Design review of the part built by this model. Coordinates are the model's own, in mm. A direction names the side the tool comes from. Round coordinates to 2 decimals unless told otherwise and drop trailing zeros. Loops run counter-clockwise (first coordinate to the right, second up) from the corner with the lowest first, then second, coordinate; pieces in that order, holes last. Notation, with made-up numbers: (69.25, 55.25) - (128.25, 55.25) arc R13 cw to (128.25, 69.25) - close; hole circle Ø5 at (45, 45). An arc over 180 degrees is marked (long way). Return JSON: item names as keys, results as strings. Group by question number.
(1) Wall thickness on L1, parallel to Y at x = 2, z = 2.1; L2, parallel to Y at x = 0.25, z = 3.8; L3, parallel to X at y = 2, z = 3.6 (3 decimals): over which ranges is each line inside the solid? List them lowest first. Write a range as [from, to].
(2) We need section D-D, the plane x = 10. Write out the cut boundary in (y, z), and give its area (3 significant figures).
(3) For faces 5 (the flat face through (4, 0, 4)), 6 (the flat face through (2.5, 0, 2)), list the 3-axis set-ups (+Z, -Z, +X, -X, +Y, -Y) from which the entire face can be reached by the end or side of a thin tool; tool diameter is ignored.
(4) We need section A-A, the plane x = 6.75. Write out the cut boundary in (y, z), and give its area (3 significant figures).
(5) The part is to be moulded in two halves that separate along X. For faces 1 (the flat face through (8, -2.5, 2)), 2 (the cylindrical face through (-3.75, -0.08, 1.97)), 3 (the flat face through (4, -3.75, 2)), 4 (the flat face through (6, -1, 2)), say which applies: pulls with the +X half, pulls with the -X half, needs draft (parallel to the pull), parting line crosses it, or undercut.
(6) We need section C-C, the plane z = 0.3. Write out the cut boundary in (x, y) (3 decimals), and give its area (3 significant figures).
(7) We need section B-B, the plane y = 0. Write out the cut boundary in (x, z) (3 decimals).
(8) Clearance check with flat-ended pins moving along their axes: pin 1 (1 mm diameter, centred on x = 9, z = 0.5, fed in from -Y); pin 2 (1.2 mm diameter, centred on y = -2, z = 1.5, fed in from +X); pin 3 (1.2 mm diameter, centred on y = 1.5, z = 1, fed in from +X). State where each tip first meets the part, or that it passes through.
from build123d import *

# Parameters (mm, degrees)
BOSS_EXTRUDE1_DEPTH = 4


with BuildPart() as part:
    # Sketch1 → Boss-Extrude1 (new body)
    with BuildSketch(Plane.XY):
        with BuildLine():
            Line((0, 3.75), (8.125, 3.75))
            ThreePointArc((8.125, 3.75), (11.875, 0), (8.125, -3.75))
            Line((8.125, -3.75), (0, -3.75))
            ThreePointArc((0, -3.75), (-3.75, 0), (0, 3.75))
        make_face()
        Polygon((8.125, 2.5), (9.125, 2.5), (9.125, 1), (10.625, 1), (10.625, -1), (9.125, -1), (9.125, -2.5), (7.125, -2.5), (7.125, -1), (5.625, -1), (5.625, 1), (7.125, 1), (7.125, 2.5), align=None, mode=Mode.SUBTRACT)
        Polygon((1, 1), (1, 2.5), (0, 2.5), (-1, 2.5), (-1, 1), (-2.5, 1), (-2.5, -1), (-1, -1), (-1, -2.5), (1, -2.5), (1, -1), (2.5, -1), (2.5, 1), align=None, mode=Mode.SUBTRACT)
    extrude(amount=BOSS_EXTRUDE1_DEPTH)


solid = part.part
Solutions:
{
 "1": {"L1": "[-3.75, -1], [1, 3.75]", "L2": "[-3.75, -2.5], [2.5, 3.75]", "L3": "[-3.172, -1], [1, 7.125], [9.125, 11.297]"},
 "2": {"outline": "(-3.25, 0) - (-1, 0) - (-1, 4) - (-3.25, 4) - close; (1, 0) - (3.25, 0) - (3.25, 4) - (1, 4) - close", "area": "18.0 mm^2"},
 "3": {"face 5": "+Z, +X, -X, +Y, -Y", "face 6": "+Z, -Z"},
 "4": {"outline": "(-3.75, 0) - (-1, 0) - (-1, 4) - (-3.75, 4) - close; (1, 0) - (3.75, 0) - (3.75, 4) - (1, 4) - close", "area": "22.0 mm^2"},
 "5": {"face 1": "undercut", "face 2": "pulls with the -X half", "face 3": "needs draft", "face 4": "undercut"},
 "6": {"outline": "(0, -3.75) - (8.125, -3.75) arc R3.75 ccw to (8.125, 3.75) - (0, 3.75) arc R3.75 ccw to start; hole (-2.5, -1) - (-1, -1) - (-1, -2.5) - (1, -2.5) - (1, -1) - (2.5, -1) - (2.5, 1) - (1, 1) - (1, 2.5) - (-1, 2.5) - (-1, 1) - (-2.5, 1) - close; hole (5.625, -1) - (7.125, -1) - (7.125, -2.5) - (9.125, -2.5) - (9.125, -1) - (10.625, -1) - (10.625, 1) - (9.125, 1) - (9.125, 2.5) - (7.125, 2.5) - (7.125, 1) - (5.625, 1) - close", "area": "73.1 mm^2"},
 "7": {"outline": "(-3.75, 0) - (-2.5, 0) - (-2.5, 4) - (-3.75, 4) - close; (2.5, 0) - (5.625, 0) - (5.625, 4) - (2.5, 4) - close; (10.625, 0) - (11.875, 0) - (11.875, 4) - (10.625, 4) - close"},
 "8": {"pin 1": "y = -3.73", "pin 2": "x = 11.6", "pin 3": "x = 11.77"}
}
